The figure shows three views and two pictorial views of one solid part (mm, origin at its lowest corner). Answer the questions. A direction names the side the tool comes from. Coordinates: 2 decimals unless noted, no trailing zeros. Order: outer loops, then holes, each group sorted by start corner. A loop starts at its lowest first (then second) coordinate and runs counter-clockwise, first axis right, second up.
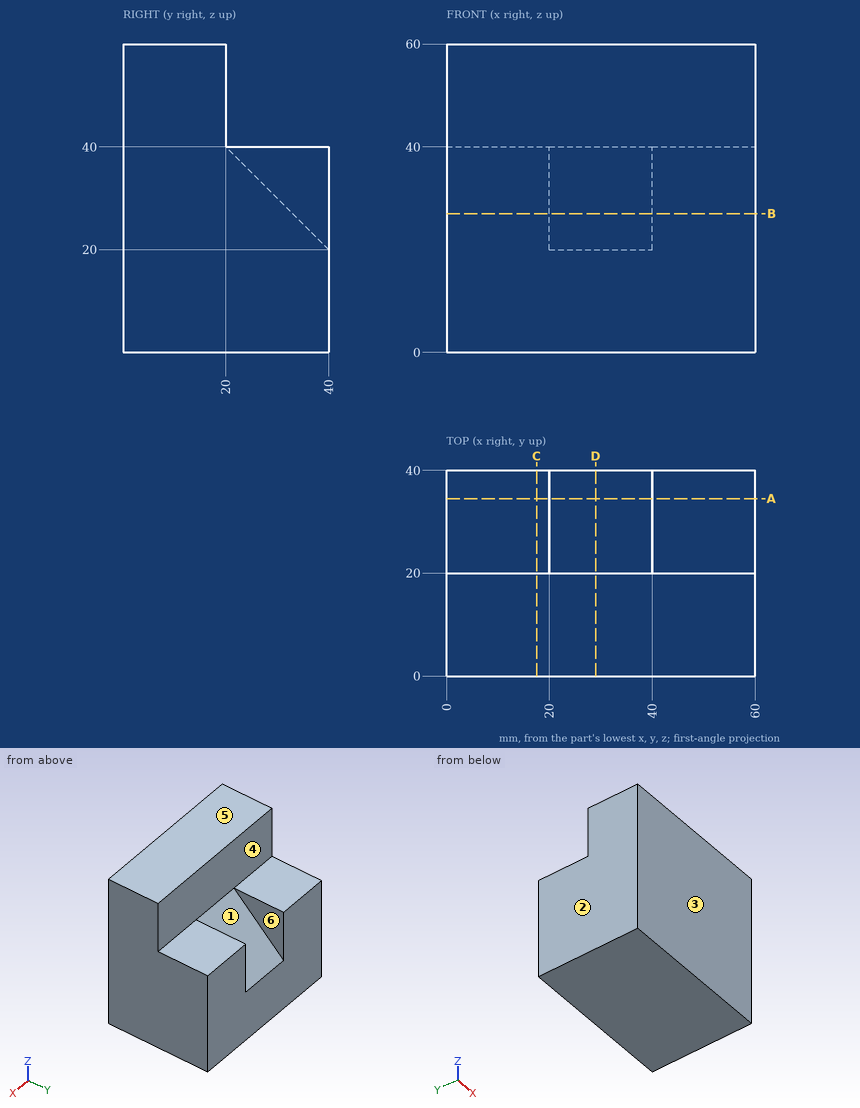
Q1. The part is cut by section B-B, the plane z = 27. Determine the outline of the cut face in (x, y).
Q2. The part is cut by section D-D, the plane x = 29. Determine the outline of the cut face in (y, z).
Q3. The part is cut by section C-C, the plane x = 17.5. Determine the outline of the cut face in (y, z).
Q4. Straight lines are drawn through the part: L1, parallel to Z at x = 9.5, y = 28; L2, parallel to Y at x = 22, z = 55; L3, parallel to Z at x = 22, y = 38.5. For each, find the intervals that lie inside material, in ascending order.
Q5. Which of the six approach directions +Z, -Z, +X, -X, +Y, -Y give full straight-line access (tool end or side, diameter ignored) to the marked faces 4, 5 and 6?
Q6. The part is cut by section A-A, the plane y = 34.5. Determine the outline of the cut face in (x, z).
Q7. Determine the mould class of the marked faces 1, 2 and 3 for opening direction X: +X half, -X half, draft (parallel to the pull), parting line (faces both ways), or undercut.
Q8. Each of these flat-tipped pins is pushed along its axis until it touches: P1, Ø10, axis at x = 29.5, z = 47, coming from the +Y side; P2, Ø22, axis at x = 47, y = 34.5, coming from the +Z side. Where does it stop, or does it pass through?
Computed values:
1. outline: (0, 0) - (60, 0) - (60, 40) - (40, 40) - (40, 33) - (20, 33) - (20, 40) - (0, 40) - close
2. outline: (0, 0) - (40, 0) - (40, 20) - (20, 40) - (20, 60) - (0, 60) - close
3. outline: (0, 0) - (40, 0) - (40, 40) - (20, 40) - (20, 60) - (0, 60) - close
4. L1: z = 0 to 40
4. L2: y = 0 to 20
4. L3: z = 0 to 21.5
5. face 4: +Z, +X, -X, +Y
5. face 5: +Z, +X, -X, +Y, -Y
5. face 6: +Z, +Y
6. outline: (0, 0) - (60, 0) - (60, 40) - (40, 40) - (40, 25.5) - (20, 25.5) - (20, 40) - (0, 40) - close
7. face 1: undercut
7. face 2: -X half
7. face 3: draft
8. P1: stops at y = 20
8. P2: stops at z = 40
